Part print with two shaded views. Sizes in mm from the minimum x, y, z corner. Round coordinates to 2 decimals unless told otherwise and drop trailing zeros. Write each loop counter-clockwise with the first axis right and the second up, starting at its lowest first coordinate (ties: lowest second). Pieces come first, ordered by that corner, then holes. Notation, with made-up numbers: (64, -10.75) - (83, -10.75) arc R9 ccw to (83, -0.75) - close; hole circle Ø8 at (28.5, 23). An arc over 180 degrees is marked (long way). Use one line per item in the form item = value. Start each with the question number.
Item 1: Pin check, flat tips, straight feed: pin 1 (2.5 mm diameter, centred on y = 2, z = 8.5, fed in from -X); pin 2 (1.1 mm diameter, centred on x = 3, y = 2, fed in from -Z) (3 decimals); pin 3 (3 mm diameter, centred on x = 1.5, y = 3.5, fed in from +Z) (3 decimals). Stop position of each tip, or through.
Item 2: Band-saw the part on B-B, the plane z = 131. List the corners of the cut face in (x, y).
Item 3: Band-saw the part on A-A, the plane x = 53.5. List the corners of the cut face in (y, z), and give its area (3 significant figures).
Item 4: Drill centre lines: L1, parallel to Z at x = 15, y = 4.4; L2, parallel to X at y = 0.95, z = 38; L3, parallel to X at y = 1.35, z = 11.5. Where is each one in solid material? Low to high.
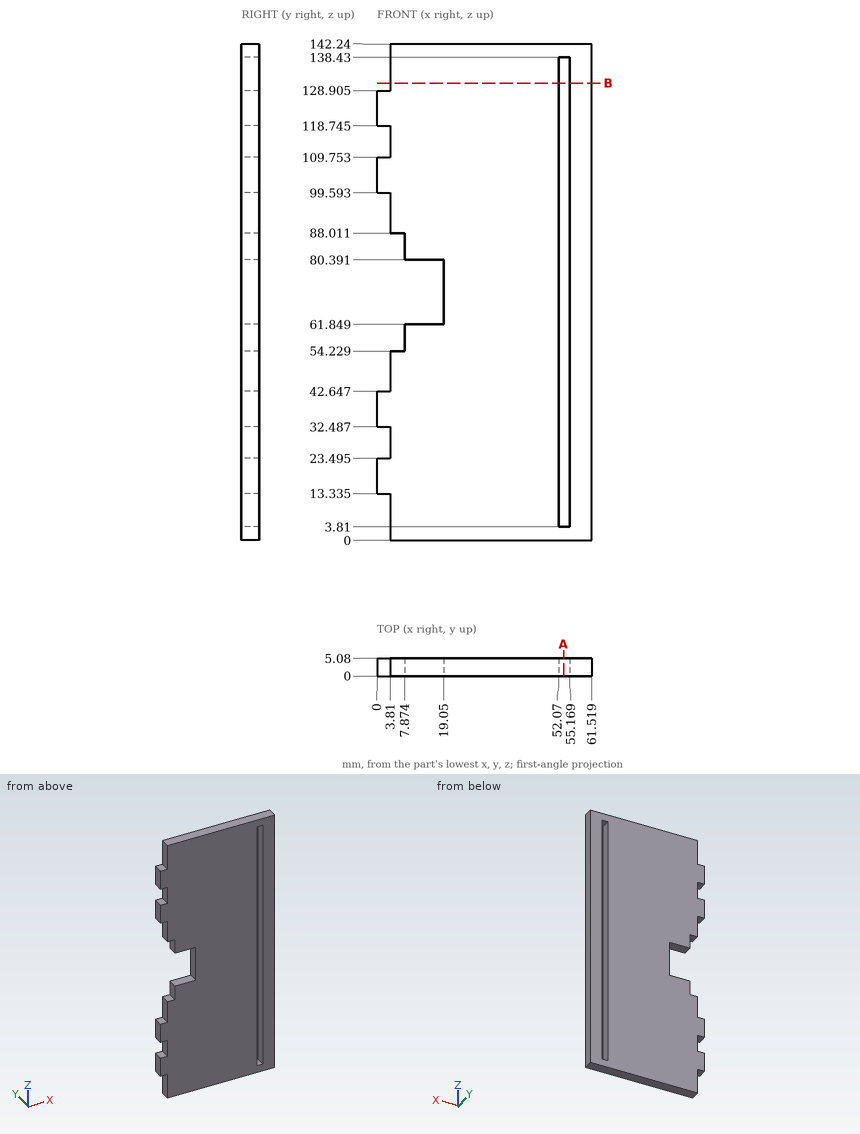
Determined:
q1.pin_1 = 3.81
q1.pin_2 = 13.335
q1.pin_3 = 128.905
q2.outline = (3.81, 0) - (52.07, 0) - (52.07, 5.08) - (3.81, 5.08) - close; (55.17, 0) - (61.52, 0) - (61.52, 5.08) - (55.17, 5.08) - close
q3.outline = (0, 0) - (5.08, 0) - (5.08, 3.81) - (0, 3.81) - close; (0, 138.43) - (5.08, 138.43) - (5.08, 142.24) - (0, 142.24) - close
q3.area = 38.7 mm²
q4.L1 = 0 to 61.85, 80.39 to 142.24
q4.L2 = 0 to 52.07, 55.17 to 61.52
q4.L3 = 3.81 to 52.07, 55.17 to 61.52
